Could you check a few things on this model? Use its own coordinates, in mm. Face numbers are marked on the shaded views. A direction names the side the tool comes from. Round coordinates to 2 decimals unless told otherwise and drop trailing zeros. Loops run counter-clockwise (first coordinate to the right, second up) from the corner with the lowest first, then second, coordinate; pieces in that order, holes last. Notation, with made-up numbers: (66, 39.25) - (80, 39.25) arc R20 ccw to (80, 55.25) - close; hole circle Ø6 at (52.25, 13). An arc over 180 degrees is marked (long way). Answer as CSV lines item,"result". Start each with the question number.
1) Suppose I cut it at B-B, the plane z = 2.5. Write out the boundary of the cut face in (x, y).
2) I'm going to push flat-ended pins straight in: pin 1 Ø2.5 at (y, z) = (-25.83, 7.79) entering from +X; pin 2 Ø4 at (x, y) = (23, 0) entering from +Z; pin 3 Ø5.5 at (x, z) = (7, 3) entering from -Y. Where does each tip first touch, or does it pass through?
3) Please list where these lines run through material, in increasing order: line 1 along Y through (x, z) = (-20, 2.8); line 2 along X through (y, z) = (-21, 4.75); line 3 along Z through (x, y) = (24, 3.5).
4) Which directions (+Z, -Z, +X, -X, +Y, -Y) give clear straight access to the entire face, cutting with the end or side of a thin tool? Please do the marked faces 5, 6 and 7.
5) We'd pull the mould along X, two halves only. Please class the marked faces 1, 2, 3 and 4: pulls with the +X half, pulls with the -X half, needs draft (parallel to the pull), parting line crosses it, or undercut.
6) Suppose I cut it at A-A, the plane y = 0. Write out the boundary of the cut face in (x, z), then the cut area to 3 significant figures.
7) Suppose I cut it at C-C, the plane y = -14. Write out the boundary of the cut face in (x, z).
8) Suppose I cut it at D-D, the plane z = 8.5. Write out the boundary of the cut face in (x, y).
```python
from build123d import *

# Parameters (mm, degrees)
BOSS_EXTRU_1_DEPTH      = 5
ESQUISSE3_R             = 1.5
BOSS_EXTRU_2_DEPTH      = 5
CONG_1_R                = 5
ENL_V_START             = -1.5
ESQUISSE4_R             = 2
ENL_V_MAT_EXTRU_1_DEPTH = 2


with BuildPart() as part:
    # Esquisse2 → Boss.-Extru.1 (new body)
    with BuildSketch(Plane.XY):
        with BuildLine():
            Line((-27.5, 5), (27.5, 5))
            ThreePointArc((27.5, 5), (29.267766953, 4.267766953), (30, 2.5))
            Line((30, 2.5), (30, -5))
            Line((30, -5), (-30, -5))
            Line((-30, -5), (-30, 2.5))
            ThreePointArc((-30, 2.5), (-29.267766953, 4.267766953), (-27.5, 5))
        make_face()
    extrude(amount=BOSS_EXTRU_1_DEPTH)

    # Esquisse3 → Boss.-Extru.2 (add)
    with BuildSketch(Plane.ZY.offset(30)):
        with BuildLine():
            ThreePointArc((0, -5), (1.419495531, -16.359810014), (5.590686777, -27.021020765))
            ThreePointArc((5.590686777, -27.021020765), (8.980460201, -28.025727757), (9.985167192, -24.635954333))
            ThreePointArc((9.985167192, -24.635954333), (6.265751924, -15.129444636), (5, -5))
            Line((5, -5), (0, -5))
        make_face()
        with Locations((7.787926985, -25.828487549)):
            Circle(ESQUISSE3_R, mode=Mode.SUBTRACT)
    boss_extru_2 = extrude(amount=-BOSS_EXTRU_2_DEPTH)

    # Symétrie1: Boss.-Extru.2 across plane
    add(boss_extru_2.mirror(Plane(origin=(0, 0, 0), x_dir=(0, 0, 1), z_dir=(1, 0, 0))))

    # Congé1
    # the kernel refuses this fillet: 5 mm, written as the material it adds along each edge
    with BuildSketch(Plane(origin=(-25, -5, 17.5), x_dir=(1, 0, 0), z_dir=(0, 0, -1))) as cong_1_piece_1_section:
        with BuildLine():
            CenterArc((CONG_1_R, CONG_1_R), CONG_1_R, 180, 90)
            Line((0, CONG_1_R), (0, 0))
            Line((0, 0), (CONG_1_R, 0))
        make_face()
    cong_1_piece_1 = extrude(amount=30, mode=Mode.PRIVATE)
    cong_1_piece_1 = cong_1_piece_1 & Plane(origin=(-24.565871858, -5, 46.164376109), x_dir=(0, 0, -1), z_dir=(-1, 0, 0)) * Cylinder(46.164376109, 80, mode=Mode.PRIVATE)
    cong_1_piece_1 = cong_1_piece_1 - Plane(origin=(-24.565871858, -5, 46.164376109), x_dir=(0, -0.4770132864696082, -0.8788960828968709), z_dir=(-1, 0, 0)) * Cylinder(41.164376109, 80, mode=Mode.PRIVATE)
    add(cong_1_piece_1)
    with BuildSketch(Plane(origin=(25, -5, 17.5), x_dir=(-1, 0, 0), z_dir=(0, 0, -1))) as cong_1_piece_2_section:
        with BuildLine():
            CenterArc((CONG_1_R, -CONG_1_R), CONG_1_R, 90, 90)
            Line((0, -CONG_1_R), (0, 0))
            Line((0, 0), (CONG_1_R, 0))
        make_face()
    cong_1_piece_2 = extrude(amount=30, mode=Mode.PRIVATE)
    cong_1_piece_2 = cong_1_piece_2 & Plane(origin=(24.565871858, -5, 46.164376109), x_dir=(0, 0, -1), z_dir=(1, 0, 0)) * Cylinder(46.164376109, 80, mode=Mode.PRIVATE)
    cong_1_piece_2 = cong_1_piece_2 - Plane(origin=(24.565871858, -5, 46.164376109), x_dir=(0, -0.4770132864696082, -0.8788960828968709), z_dir=(1, 0, 0)) * Cylinder(41.164376109, 80, mode=Mode.PRIVATE)
    add(cong_1_piece_2)

    # Esquisse4 → Enlèv. mat.-Extru.1 (cut)
    with BuildSketch(Plane(origin=(0, 0, 0), x_dir=(-1, 0, 0), z_dir=(0, 0, -1)).offset(ENL_V_START)):
        with Locations((-20, 0)):
            Circle(ESQUISSE4_R)
        with Locations((20, 0)):
            Circle(ESQUISSE4_R)
    extrude(amount=-ENL_V_MAT_EXTRU_1_DEPTH, mode=Mode.SUBTRACT)


solid = part.part
```
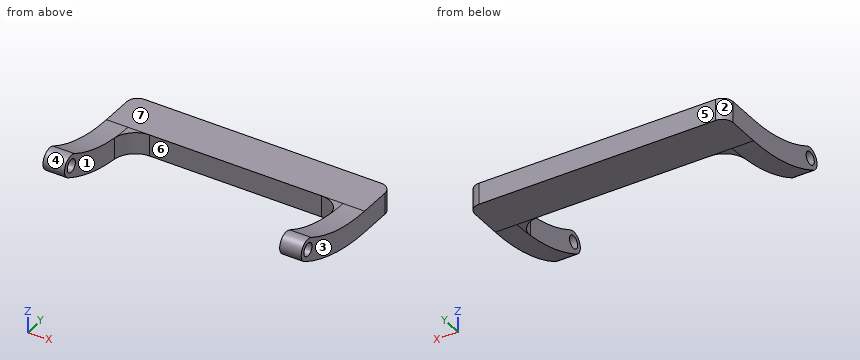
Filled sheet:
1,outline,"(-30, -19.99) - (-25, -19.99) - (-25, -10) arc R5 cw to (-20, -5) - (20, -5) arc R5 cw to (25, -10) - (25, -19.99) - (30, -19.99) - (30, 2.5) arc R2.5 ccw to (27.5, 5) - (-27.5, 5) arc R2.5 ccw to (-30, 2.5) - close; hole circle Ø4 at (-20, 0); hole circle Ø4 at (20, 0)"
2,pin 1,"through"
2,pin 2,"z = 5"
2,pin 3,"y = -5"
3,line 1,"-5 to -2, 2 to 5"
3,line 2,"-30 to -25, 25 to 30"
3,line 3,"0 to 5"
4,face 5,"+Z, -Z, +X, -X, +Y"
4,face 6,"+Z, -Z, -Y"
4,face 7,"+Z, +X, -X, +Y"
5,face 1,"undercut"
5,face 2,"pulls with the -X half"
5,face 3,"pulls with the +X half"
5,face 4,"needs draft"
6,outline,"(-30, 0) - (30, 0) - (30, 5) - (-30, 5) - close; hole (-22, 1.5) - (-18, 1.5) - (-18, 3.5) - (-22, 3.5) - close; hole (18, 1.5) - (22, 1.5) - (22, 3.5) - (18, 3.5) - close"
6,area,"284 mm²"
7,outline,"(-30, 0.89) - (-25, 0.89) - (-25, 6) - (-30, 6) - close; (25, 0.89) - (30, 0.89) - (30, 6) - (25, 6) - close"
8,outline,"(-30, -28.22) - (-25, -28.22) - (-25, -27.15) - (-30, -27.15) - close; (-30, -24.51) - (-25, -24.51) - (-25, -21.61) - (-30, -21.61) - close; (25, -28.22) - (30, -28.22) - (30, -27.15) - (25, -27.15) - close; (25, -24.51) - (30, -24.51) - (30, -21.61) - (25, -21.61) - close"
